Geometry: see drawing. Coordinates: mm, zero at the bounding-box minimum. A direction names the side the tool comes from. Coordinates: 2 decimals unless noted, no trailing zeros. Write each loop counter-clockwise with the first axis right and the second up, starting at its lowest first coordinate (ties: lowest second). Pieces come first, ordered by that corner, then holes.
1) Set-up query: the marked faces 1 and 2. Return all of +Z, -Z, +X, -X, +Y, -Y with unobstructed straight access to the full face (end or side cutting, diameter ignored); none if empty.
2) Pin query (flat end, axial travel): pin 1 Ø5 at (x, y) = (115.5, 84.5) entering from +Z; pin 2 Ø1.2 at (y, z) = (91, 14) entering from +X; pin 3 Ø7 at (x, y) = (9, 64.5) entering from -Z. Return the tip coordinate at first contact, or that it passes through.
3) Section query B-B (z = 5). Output: boundary loops of the cut face in (x, y).
4) Line query: L1, parallel to Y at x = 5, z = 67; L2, parallel to X at y = 30, z = 35.5. Output: solid intervals per line, ascending.
5) Section query C-C (y = 90). Output: boundary loops of the cut face in (x, z).
6) Section query A-A (x = 5). Output: boundary loops of the cut face in (y, z).
7) Section query D-D (y = 31.5). Output: boundary loops of the cut face in (x, z), then the cut area to 3 significant figures.
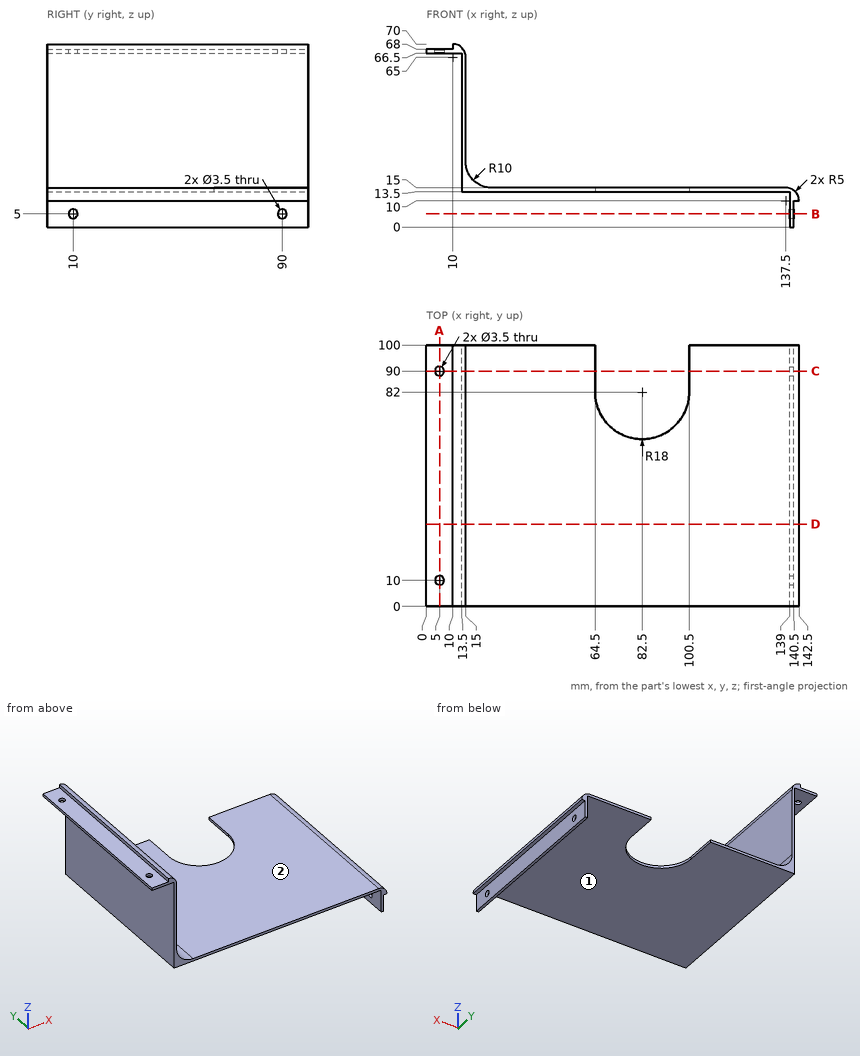
Answer:
1. face 1: -Z, -X, +Y, -Y
1. face 2: +Z, +X, +Y, -Y
2. pin 1: stops at z = 15
2. pin 2: stops at x = 141.17
2. pin 3: stops at z = 66.5
3. outline: (139, 0) - (140.5, 0) - (140.5, 8.25) - (139, 8.25) - close; (139, 11.75) - (140.5, 11.75) - (140.5, 88.25) - (139, 88.25) - close; (139, 91.75) - (140.5, 91.75) - (140.5, 100) - (139, 100) - close
4. L1: y = 0 to 8.25, 11.75 to 88.25, 91.75 to 100
4. L2: x = 13.5 to 15
5. outline: (0, 66.5) - (3.25, 66.5) - (3.25, 68) - (0, 68) - close; (6.75, 66.5) - (13.5, 66.5) - (13.5, 13.5) - (64.5, 13.5) - (64.5, 15) - (25, 15) arc R10 cw to (15, 25) - (15, 65) arc R5 ccw to (10, 70) - (10, 68) - (6.75, 68) - close; (100.5, 13.5) - (139, 13.5) - (139, 6.75) - (140.5, 6.75) - (140.5, 10) - (142.5, 10) arc R5 ccw to (137.5, 15) - (100.5, 15) - close; (139, 0) - (140.5, 0) - (140.5, 3.25) - (139, 3.25) - close
6. outline: (0, 66.5) - (8.25, 66.5) - (8.25, 68) - (0, 68) - close; (11.75, 66.5) - (88.25, 66.5) - (88.25, 68) - (11.75, 68) - close; (91.75, 66.5) - (100, 66.5) - (100, 68) - (91.75, 68) - close
7. outline: (0, 66.5) - (13.5, 66.5) - (13.5, 13.5) - (139, 13.5) - (139, 0) - (140.5, 0) - (140.5, 10) - (142.5, 10) arc R5 ccw to (137.5, 15) - (25, 15) arc R10 cw to (15, 25) - (15, 65) arc R5 ccw to (10, 70) - (10, 68) - (0, 68) - close
7. area: 341 mm2
